Geometry: final body of the model. Coordinates: model frame, mm. A direction names the side the tool comes from. Round coordinates to 2 decimals unless told otherwise and drop trailing zeros. Order: outer loops, then holes, each group sorted by start corner. A loop starts at its lowest first (then second) coordinate and runs counter-clockwise, first axis right, second up. Notation, with made-up numbers: M -11,25.25 L 25,25.25 A19 ccw 25,47.25 Z; hole C -4.75,60.25 d2. An arc over 180 degrees is marked long. Put each result on its own line as item: value. Start each with the question number.
1) Section A-A, the plane z = 150.5. Return loops of the section in (x, y), then the cut area to 3 significant figures.
2) Section C-C, the plane x = 11. Return loops of the section in (y, z), then the cut area to 3 significant figures.
3) Access query for faces 1 (the flat face through (22, 6.35, 157)), 2 (the flat face through (19, 0, 138)), 3 (the flat face through (22, 3, 38.1)), 4 (the flat face through (6.35, 3, 263)). Directions: +Z, -Z, +X, -X, +Y, -Y. A direction counts if a zero-diameter tool reaches every point of the face in a straight line with its end or side. Return the directions, or none.
4) Section B-B, the plane y = 20.5. Return loops of the section in (x, z).
5) First-contact query: P1, Ø19, axis at y = 23.5, z = 64.5, coming from the +X side; P2, Ø7, axis at y = 4, z = 266, coming from the -X side; P3, Ø5, axis at x = 22, y = 3.5, coming from the -Z side. Flat tips, straight axial feed; report the tip coordinate or a pass-through.
6) Material intervals for probe 1 along X at (y, z) = (23, 55.5); probe 2 along Z at (x, y) = (3, 10), sorted ascending. Write a range as [from, to].
from build123d import *

# Parameters (mm, degrees)
BOSS_EXTRUDE1_DEPTH = 279.4
SKETCH2_W           = 31.75
SKETCH2_H           = 38.1
CUT_EXTRUDE1_DEPTH  = 6.35
SKETCH3_W           = 31.75
SKETCH3_H           = 38.1
CUT_EXTRUDE2_DEPTH  = 39.1
CUT_EXTRUDE3_DEPTH  = 39.1


with BuildPart() as part:
    # Sketch1 → Boss-Extrude1 (new body)
    with BuildSketch(Plane.XY):
        Polygon((0, 0), (0, 38.1), (6.35, 38.1), (6.35, 6.35), (38.1, 6.35), (38.1, 0), align=None)
    extrude(amount=BOSS_EXTRUDE1_DEPTH)

    # Sketch2 → Cut-Extrude1 (cut)
    with BuildSketch(Plane.ZY):
        with Locations((263.525, 19.05)):
            Rectangle(SKETCH2_W, SKETCH2_H)
    extrude(amount=-CUT_EXTRUDE1_DEPTH, mode=Mode.SUBTRACT)

    # Sketch3 → Cut-Extrude2 (cut, through all)
    with BuildSketch(Plane.XZ):
        with Locations((22.225, 19.05)):
            Rectangle(SKETCH3_W, SKETCH3_H)
    extrude(amount=-CUT_EXTRUDE2_DEPTH, mode=Mode.SUBTRACT)

    # Sketch4 → Cut-Extrude3 (cut, through all)
    with BuildSketch(Plane.ZY):
        Polygon((0, 38.1), (0, 25.4), (12.7, 38.1), align=None)
    extrude(amount=-CUT_EXTRUDE3_DEPTH, mode=Mode.SUBTRACT)


solid = part.part
Result sheet:
1. outline: M 0,0 L 38.1,0 L 38.1,6.35 L 6.35,6.35 L 6.35,38.1 L 0,38.1 Z
1. area: 444 mm2
2. outline: M 0,38.1 L 6.35,38.1 L 6.35,279.4 L 0,279.4 Z
2. area: 1,530 mm2
3. face 1: +Z, -Z, +X, +Y
3. face 2: +Z, -Z, +X, -X, -Y
3. face 3: -Z, +X, +Y, -Y
3. face 4: +Z, -X, +Y, -Y
4. outline: M 0,0 L 6.35,0 L 6.35,247.65 L 0,247.65 Z
5. P1: stops at x = 6.35
5. P2: stops at x = 6.35
5. P3: stops at z = 38.1
6. probe 1: x = [0, 6.35]
6. probe 2: z = [0, 247.65]
